from build123d import *

# Parameters (mm, degrees)
BOSS_EXTRUDE1_DEPTH = 20
BOSS_EXTRUDE2_DEPTH = 12.7
BOSS_EXTRUDE3_DEPTH = 2
SKETCH4_W           = 52.357488091
SKETCH4_H           = 8.89
CUT_EXTRUDE1_DEPTH  = 22


with BuildPart() as part:
    # Sketch1 → Boss-Extrude1 (new body)
    with BuildSketch(Plane(origin=(0, 0, 0), x_dir=(1, 0, 0), z_dir=(0, 1, 0))):
        with BuildLine():
            Line((-18.32, 0), (-18.32, 2.075569274))
            Line((-18.32, 2.075569274), (-18.32, 10.32))
            Line((-18.32, 10.32), (-25, 10.32))
            Line((-25, 10.32), (-25, 13.32))
            Line((-25, 13.32), (-13.32, 13.32))
            Line((-13.32, 13.32), (-13.32, 0))
            ThreePointArc((-13.32, 0), (0, -13.32), (13.32, 0))
            Line((13.32, 0), (13.32, 13.32))
            Line((13.32, 13.32), (25, 13.32))
            Line((25, 13.32), (25, 10.32))
            Line((25, 10.32), (18.32, 10.32))
            Line((18.32, 10.32), (18.32, 1.685292353))
            Line((18.32, 1.685292353), (18.32, 0))
            ThreePointArc((18.32, 0), (0, -18.32), (-18.32, 0))
        make_face()
    extrude(amount=BOSS_EXTRUDE1_DEPTH)

    # Sketch2 → Boss-Extrude2 (add)
    with BuildSketch(Plane(origin=(0, 20, 0), x_dir=(1, 0, 0), z_dir=(0, 1, 0))):
        with BuildLine():
            Line((-18.32, 10.32), (-18.32, 0))
            ThreePointArc((-18.32, 0), (0, -18.32), (18.32, 0))
            Line((18.32, 0), (18.32, 10.32))
            Line((18.32, 10.32), (25, 10.32))
            Line((25, 10.32), (25, 13.32))
            Line((25, 13.32), (13.32, 13.32))
            Line((13.32, 13.32), (13.32, 0))
            ThreePointArc((13.32, 0), (0, -13.32), (-13.32, 0))
            Line((-13.32, 0), (-13.32, 13.32))
            Line((-13.32, 13.32), (-25, 13.32))
            Line((-25, 13.32), (-25, 10.32))
            Line((-25, 10.32), (-18.32, 10.32))
        make_face()
    extrude(amount=BOSS_EXTRUDE2_DEPTH)

    # Sketch3 → Boss-Extrude3 (add)
    with BuildSketch(Plane(origin=(0, 32.7, 0), x_dir=(1, 0, 0), z_dir=(0, 1, 0))):
        with BuildLine():
            Line((-10.82, 13.32), (-13.32, 13.32))
            Line((-13.32, 13.32), (-13.32, 0))
            ThreePointArc((-13.32, 0), (0, -13.32), (13.32, 0))
            Line((13.32, 0), (13.32, 13.32))
            Line((13.32, 13.32), (10.82, 13.32))
            Line((10.82, 13.32), (10.82, 0))
            ThreePointArc((10.82, 0), (0, -10.82), (-10.82, 0))
            Line((-10.82, 0), (-10.82, 13.32))
        make_face()
        with BuildLine():
            Line((-25, 13.32), (-25, 10.32))
            Line((-25, 10.32), (-18.32, 10.32))
            Line((-18.32, 10.32), (-18.32, 0))
            ThreePointArc((-18.32, 0), (0, -18.32), (18.32, 0))
            Line((18.32, 0), (18.32, 10.32))
            Line((18.32, 10.32), (25, 10.32))
            Line((25, 10.32), (25, 13.32))
            Line((25, 13.32), (13.32, 13.32))
            Line((13.32, 13.32), (13.32, 0))
            ThreePointArc((13.32, 0), (0, -13.32), (-13.32, 0))
            Line((-13.32, 0), (-13.32, 13.32))
            Line((-13.32, 13.32), (-25, 13.32))
        make_face()
    extrude(amount=BOSS_EXTRUDE3_DEPTH)

    # Sketch4 → Cut-Extrude1 (cut, symmetric)
    with BuildSketch(Plane.XY):
        with Locations((1.178744046, 4.445)):
            Rectangle(SKETCH4_W, SKETCH4_H)
    extrude(amount=CUT_EXTRUDE1_DEPTH, both=True, mode=Mode.SUBTRACT)


solid = part.part
The listing builds one solid part. Answer for the finished solid, in the listing's coordinates (mm). A direction names the side the tool comes from. Coordinates: 2 decimals unless noted, no trailing zeros. Loops run counter-clockwise (first coordinate to the right, second up) from the corner with the lowest first, then second, coordinate; pieces in that order, holes last.
1) A tool of negligible diameter and unlimited length cuts with its end or side. For faces 1 (the face through (-22, 22, -10.32)), 2 (the face through (22, 22, -10.32)), 3 (the face through (-4, 8.89, 13)), 4 (the face through (0.293, 20.628, 13.317)), 5 (the face through (10.82, 34, -7)), from which of +Z, -Z, +X, -X, +Y, -Y can it reach the whole face along a straight path? Write none if from no direction.
2) Find section A-A on z = -7. Write down the section's boundary in (x, y).
3) Find section D-D on z = 3. Write down the section's boundary in (x, y).
4) Determine the mould class of faces 6 (the face through (18.32, 22, -5)), 7 (the face through (-5.9, 34.7, 9.3)), 8 (the face through (13.32, 21, -7)) for opening direction X: pulls with the +X half, pulls with the -X half, needs draft (parallel to the pull), parting line crosses it, or undercut.
5) Find section C-C on x = 0. Write down the section's boundary in (y, z), then the cut area to 3 significant figures.
6) Flat-ended cylindrical pins translate along their axes: pin 1 Ø3.5 at (x, y) = (21.5, 25.5) entering from +Z; pin 2 Ø1.5 at (x, z) = (-9.5, 6) entering from -Y; pin 3 Ø4 at (y, z) = (24.5, -5.5) entering from -X. Find the tip coordinate at first contact, or state that the pin passes through.
7) Find section B-B on y = 18.75. Write down the section's boundary in (x, z).
8) Find the intervals of material crossed by L1, parallel to X at y = 13.75, z = -11; L2, parallel to X at y = 32, z = -9; L3, parallel to Z at x = 22.5, y = 23.75, in increasing order.
Values:
1. face 1: +Z, -X, +Y, -Y
1. face 2: +Z, +X, +Y, -Y
1. face 3: +Z, -Z, +X, -X, -Y
1. face 4: -Z, -Y
1. face 5: -Z, +Y, -Y
2. outline: (-18.32, 8.89) - (-13.32, 8.89) - (-13.32, 32.7) - (-10.82, 32.7) - (-10.82, 34.7) - (-18.32, 34.7) - close; (10.82, 32.7) - (13.32, 32.7) - (13.32, 8.89) - (18.32, 8.89) - (18.32, 34.7) - (10.82, 34.7) - close
3. outline: (-18.07, 8.89) - (-12.98, 8.89) - (-12.98, 32.7) - (-10.4, 32.7) - (-10.4, 34.7) - (-18.07, 34.7) - close; (10.4, 32.7) - (12.98, 32.7) - (12.98, 8.89) - (18.07, 8.89) - (18.07, 34.7) - (10.4, 34.7) - close
4. face 6: pulls with the +X half
4. face 7: needs draft
4. face 8: undercut
5. outline: (8.89, 13.32) - (32.7, 13.32) - (32.7, 10.82) - (34.7, 10.82) - (34.7, 18.32) - (8.89, 18.32) - close
5. area: 134 mm2
6. pin 1: stops at z = -10.32
6. pin 2: stops at y = 32.7
6. pin 3: stops at x = -18.32
7. outline: (-25, -13.32) - (-13.32, -13.32) - (-13.32, 0) arc R13.32 cw to (13.32, 0) - (13.32, -13.32) - (25, -13.32) - (25, -10.32) - (18.32, -10.32) - (18.32, 0) arc R18.32 ccw to (-18.32, 0) - (-18.32, -10.32) - (-25, -10.32) - close
8. L1: x = -25 to -13.32, 13.32 to 25
8. L2: x = -18.32 to -13.32, 13.32 to 18.32
8. L3: z = -13.32 to -10.32
